Part model, mm, in its own coordinate system. A direction names the side the tool comes from. Coordinates: 2 decimals unless noted, no trailing zeros. Loops run counter-clockwise (first coordinate to the right, second up) from the corner with the lowest first, then second, coordinate; pieces in that order, holes last. Notation, with made-up numbers: M 25.25,77.25 L 82.25,77.25 A25 cw 82.25,90.25 Z; hole C 40.25,7.25 d2. An arc over 180 degrees is marked long. Use CSV: the item, a comma, the result in double quotes. Start each with the question number.
from build123d import *

# Parameters (mm, degrees)
SKETCH1_W           = 50.8
SKETCH1_H           = 50.8
BOSS_EXTRUDE1_DEPTH = 6.35
FILLET1_R           = 6.35
BOSS_EXTRUDE2_START = 19.05
BOSS_EXTRUDE2_DEPTH = 19.05
SKETCH5_W           = 50.8
SKETCH5_H           = 50.8
BOSS_EXTRUDE3_DEPTH = 6.35
FILLET2_R           = 6.35
SKETCH6_R           = 3.175
BOSS_EXTRUDE4_DEPTH = 12.7
BOSS_EXTRUDE5_DEPTH = 19.05


with BuildPart() as part:
    # Sketch1 → Boss-Extrude1 (new body)
    with BuildSketch(Plane(origin=(0, 0, 0), x_dir=(1, 0, 0), z_dir=(0, 1, 0))):
        with Locations((25.4, 25.4)):
            Rectangle(SKETCH1_W, SKETCH1_H)
    extrude(amount=BOSS_EXTRUDE1_DEPTH)

    # Fillet1
    fillet1_edges = [part.edges().sort_by_distance(p)[0] for p in [
        (0, 3.175, -50.8),
        (50.8, 3.175, -50.8),
        (50.8, 3.175, 0),
        (0, 3.175, 0),
    ]]
    fillet(fillet1_edges, radius=FILLET1_R)

    # Sketch3 → Boss-Extrude2 (add)
    with BuildSketch(Plane(origin=(0, 6.35, 0), x_dir=(1, 0, 0), z_dir=(0, 1, 0)).offset(BOSS_EXTRUDE2_START)):
        with BuildLine():
            Line((11.43, 48.26), (39.37, 48.26))
            ThreePointArc((39.37, 48.26), (48.940128061, 48.940128061), (48.26, 39.37))
            Line((48.26, 39.37), (48.26, 11.43))
            ThreePointArc((48.26, 11.43), (48.940128061, 1.859871939), (39.37, 2.54))
            Line((39.37, 2.54), (11.43, 2.54))
            ThreePointArc((11.43, 2.54), (1.859871939, 1.859871939), (2.54, 11.43))
            Line((2.54, 11.43), (2.54, 39.37))
            ThreePointArc((2.54, 39.37), (1.859871939, 48.940128061), (11.43, 48.26))
        make_face()
    extrude(amount=-BOSS_EXTRUDE2_DEPTH)

    # Sketch5 → Boss-Extrude3 (add)
    with BuildSketch(Plane(origin=(0, 25.4, 0), x_dir=(1, 0, 0), z_dir=(0, 1, 0))):
        with Locations((25.4, 25.4)):
            Rectangle(SKETCH5_W, SKETCH5_H)
    extrude(amount=BOSS_EXTRUDE3_DEPTH)

    # Fillet2
    fillet2_edges = [part.edges().sort_by_distance(p)[0] for p in [
        (50.8, 28.575, -50.8),
        (0, 28.575, -50.8),
        (50.8, 28.575, 0),
        (0, 28.575, 0),
    ]]
    fillet(fillet2_edges, radius=FILLET2_R - 0.0001)  # a hair under: the kernel refuses the full size

    # Sketch6 → Boss-Extrude4 (add)
    with BuildSketch(Plane(origin=(0, 31.75, 0), x_dir=(1, 0, 0), z_dir=(0, 1, 0))):
        with Locations(Location((25.4, 25.4, 0), (0, 0, 270))):
            Circle(SKETCH6_R)
    extrude(amount=BOSS_EXTRUDE4_DEPTH)

    # Sketch7 → Boss-Extrude5 (add)
    with BuildSketch(Plane(origin=(0, 44.45, 0), x_dir=(1, 0, 0), z_dir=(0, 1, 0))):
        with BuildLine():
            Line((28.575, 26.035), (28.575, 24.765))
            Line((28.575, 24.765), (26.854967783, 24.765))
            ThreePointArc((26.854967783, 24.765), (23.8125, 25.4), (26.854967783, 26.035))
            Line((26.854967783, 26.035), (28.575, 26.035))
        make_face()
    extrude(amount=BOSS_EXTRUDE5_DEPTH)


solid = part.part
1. Slice it at A-A, the plane y = 16.5. List the corners of the cut face in (x, z).
2. Two-plate mould, pull along X, no slides. Class faces 1 (the face through (25, 25.4, -50)), 2 (the face through (48.89, 28.62, -1.81)), 3 (the face through (25, 29, -50.8)), 4 (the face through (25, 6.35, -1)): pulls with the +X half, pulls with the -X half, needs draft (parallel to the pull), parting line crosses it, or undercut.
3. Wall check: probe 1 along Y at (x, z) = (48.5, -12.5); probe 2 along Y at (x, z) = (6, -18); probe 3 along X at (y, z) = (11.5, -20.5). Give the ranges that are in metal, low to high.
4. Slice it at D-D, the plane x = 13.5. List the corners of the cut face in (y, z), and give its area (3 significant figures).
5. Slice it at C-C, the plane z = -20. List the corners of the cut face in (x, y), and give its area (3 significant figures).
6. Tool access for faces 5 (the face through (28, 54, -24.765)), 6 (the face through (50, 6.35, -26)), 7 (the face through (2.54, 16, -25)), 8 (the face through (25, 6.35, -50)), 9 (the face through (25, 3, -50.8)): list every direction of +Z, -Z, +X, -X, +Y, -Y with a clear straight run to the whole face (end or side of a thin tool).
7. Pin check, flat tips, straight feed: pin 1 (6 mm diameter, centred on x = 13.5, y = 19, fed in from +Z); pin 2 (0.9 mm diameter, centred on x = 28, y = 56, fed in from +Z) (3 decimals); pin 3 (1.3 mm diameter, centred on x = 1, z = -25, fed in from +Y). Stop position of each tip, or through.
Found:
1,outline,"M 2.54,-39.37 A6.35 ccw long 11.43,-48.26 L 39.37,-48.26 A6.35 ccw long 48.26,-39.37 L 48.26,-11.43 A6.35 ccw long 39.37,-2.54 L 11.43,-2.54 A6.35 ccw long 2.54,-11.43 Z"
2,face 1,"undercut"
2,face 2,"pulls with the +X half"
2,face 3,"needs draft"
2,face 4,"undercut"
3,probe 1,"0 to 6.35, 25.4 to 31.75"
3,probe 2,"0 to 31.75"
3,probe 3,"2.54 to 48.26"
4,outline,"M 0,-50.8 L 6.35,-50.8 L 6.35,-48.26 L 25.4,-48.26 L 25.4,-50.8 L 31.75,-50.8 L 31.75,0 L 25.4,0 L 25.4,-2.54 L 6.35,-2.54 L 6.35,0 L 0,0 Z"
4,area,"1,520 mm^2"
5,outline,"M 0,0 L 50.8,0 L 50.8,6.35 L 48.26,6.35 L 48.26,25.4 L 50.8,25.4 L 50.8,31.75 L 0,31.75 L 0,25.4 L 2.54,25.4 L 2.54,6.35 L 0,6.35 Z"
5,area,"1,520 mm^2"
6,face 5,"+Z, +X, +Y"
6,face 6,"+X"
6,face 7,"-X"
6,face 8,"-Z"
6,face 9,"-Z, +X, -X, +Y, -Y"
7,pin 1,"z = -1.54"
7,pin 2,"z = -24.765"
7,pin 3,"y = 31.75"
